from build123d import *

# Parameters (mm, degrees)
F1_DEPTH = 3.175


with BuildPart() as f1:
    # F0 (on Front) → F1 (new body)
    with BuildSketch(Plane.XZ):
        with BuildLine():
            ThreePointArc((18.1003854029, 25.9293170253), (27.7354169074, 14.7579941641), (31.2024073118, 0.4188078519))
            ThreePointArc((31.2024073118, 0.4188078519), (15.6747583451, -26.6663225741), (-15.5443153352, -26.9519992705))
            Line((-15.5443153352, -26.9519992705), (-17.4479872613, -28.6275453194))
            ThreePointArc((-17.4479872613, -28.6275453194), (16.7522947844, -28.9206845921), (33.9376170858, 0.6497384695))
            ThreePointArc((33.9376170858, 0.6497384695), (30.1518596131, 16.2494630696), (19.6368196433, 28.3786551975))
            Line((19.6368196433, 28.3786551975), (18.1003854029, 25.9293170253))
        make_face()
        with BuildLine():
            ThreePointArc((16.3881498341, 27.0734219148), (17.253653438, 26.5154160266), (18.1003854029, 25.9293170253))
            Line((18.1003854029, 25.9293170253), (19.6368196433, 28.3786551975))
            ThreePointArc((19.6368196433, 28.3786551975), (18.8174924383, 28.9438406682), (17.9819876939, 29.4848245007))
            Line((17.9819876939, 29.4848245007), (16.3881498341, 27.0734219148))
        make_face()
        with BuildLine():
            Line((-17.4479872613, -28.6275453194), (-15.5443153352, -26.9519992705))
            ThreePointArc((-15.5443153352, -26.9519992705), (-16.2151958858, -26.5645395925), (-16.8763088681, -26.1606394314))
            Line((-16.8763088681, -26.1606394314), (-18.7192165135, -27.8357967551))
            ThreePointArc((-18.7192165135, -27.8357967551), (-18.0879575097, -28.2386644121), (-17.4479872613, -28.6275453194))
        make_face()
        with BuildLine():
            ThreePointArc((17.9819876939, 29.4848245007), (18.8174924383, 28.9438406682), (19.6368196433, 28.3786551975))
            Line((19.6368196433, 28.3786551975), (33.8907018304, 51.1017739773))
            Line((33.8907018304, 51.1017739773), (14.0615815229, 31.5986632111))
            ThreePointArc((14.0615815229, 31.5986632111), (14.88706319, 31.2075763768), (15.7017518794, 30.7944768319))
            Line((15.7017518794, 30.7944768319), (25.0723678619, 40.2122400701))
            Line((25.0723678619, 40.2122400701), (17.9819876939, 29.4848245007))
        make_face()
        with BuildLine():
            Line((-35.7383415103, -44.7260811925), (-17.4479872613, -28.6275453194))
            ThreePointArc((-17.4479872613, -28.6275453194), (-18.0879575097, -28.2386644121), (-18.7192165135, -27.8357967551))
            Line((-18.7192165135, -27.8357967551), (-27.7228504419, -36.0198765993))
            Line((-27.7228504419, -36.0198765993), (-20.4711550552, -26.6101538588))
            ThreePointArc((-20.4711550552, -26.6101538588), (-21.1322326485, -26.1033010296), (-21.7807070785, -25.5804202701))
            Line((-21.7807070785, -25.5804202701), (-35.7383415103, -44.7260811925))
        make_face()
        with BuildLine():
            ThreePointArc((11.8378918102, 29.4115330659), (12.702739818, 29.0376137231), (13.5559743104, 28.6379030117))
            Line((13.5559743104, 28.6379030117), (15.7017518794, 30.7944768319))
            ThreePointArc((15.7017518794, 30.7944768319), (14.88706319, 31.2075763768), (14.0615815229, 31.5986632111))
            Line((14.0615815229, 31.5986632111), (11.8378918102, 29.4115330659))
        make_face()
        with BuildLine():
            Line((-20.4711550552, -26.6101538588), (-19.0004213571, -24.7017454678))
            ThreePointArc((-19.000421357, -24.7017454678), (-19.6857633723, -24.1734886316), (-20.3562825888, -23.6265398743))
            Line((-20.3562825888, -23.6265398743), (-21.7807070785, -25.5804202701))
            ThreePointArc((-21.7807070785, -25.5804202701), (-21.1322326485, -26.1033010296), (-20.4711550552, -26.6101538588))
        make_face()
        with BuildLine():
            ThreePointArc((-20.3562825888, -23.6265398743), (-27.0142720371, 16.7048556324), (11.8378918102, 29.4115330659))
            Line((11.8378918102, 29.4115330659), (14.0615815229, 31.5986632111))
            ThreePointArc((14.0615815229, 31.5986632111), (-28.9318907936, 18.7255261755), (-21.7807070785, -25.5804202701))
            Line((-21.7807070785, -25.5804202701), (-20.3562825888, -23.6265398743))
        make_face()
        with BuildLine():
            Line((-5.9004323557, 9.0836035088), (13.5559743104, 28.6379030117))
            ThreePointArc((13.5559743104, 28.6379030117), (12.702739818, 29.0376137231), (11.8378918102, 29.4115330659))
            Line((11.8378918102, 29.4115330659), (-11.5615911782, 6.3967597671))
            Line((-11.5615911782, 6.3967597671), (-3.1656639185, 7.3638306931))
            Line((-3.1656639185, 7.3638306931), (-20.9245868027, -14.5271206275))
            Line((-20.9245868027, -14.5271206275), (-12.4407447875, -12.7688115463))
            Line((-12.4407447875, -12.7688115463), (-20.3562825888, -23.6265398743))
            ThreePointArc((-20.3562825888, -23.6265398743), (-19.6857633723, -24.1734886316), (-19.000421357, -24.7017454678))
            Line((-19.0004213571, -24.7017454678), (-7.2250561789, -9.4221569598))
            Line((-7.2250561789, -9.4221569598), (-15.4455099255, -11.0584562644))
            Line((-15.4455099255, -11.0584562644), (1.6187507426, 9.8238335922))
            Line((1.6187507426, 9.8238335922), (-5.9004323557, 9.0836035088))
        make_face()
        with BuildLine():
            Line((14.2855551094, 19.8478270322), (18.1003854029, 25.9293170253))
            ThreePointArc((18.1003854029, 25.9293170253), (17.253653438, 26.5154160266), (16.3881498341, 27.0734219148))
            Line((16.3881498341, 27.0734219148), (10.034003295, 17.4598935992))
            Line((10.034003295, 17.4598935992), (18.7998898327, 17.4598935992))
            Line((18.7998898327, 17.4598935992), (5.6315795518, 0))
            Line((5.6315795518, 0), (11.9040580466, 0))
            Line((11.9040580466, 0), (-16.8763088681, -26.1606394314))
            ThreePointArc((-16.8763088681, -26.1606394314), (-16.2151958858, -26.5645395925), (-15.5443153352, -26.9519992705))
            Line((-15.5443153352, -26.9519992705), (17.4505114555, 2.0889036823))
            Line((17.4505114555, 2.0889036823), (10.2414432913, 2.0889036823))
            Line((10.2414432913, 2.0889036823), (23.1650173664, 19.8478270322))
            Line((23.1650173664, 19.8478270322), (14.2855551094, 19.8478270322))
        make_face()
    extrude(amount=F1_DEPTH)


solid = f1.part
Can you work these out from the model? Positions are in its coordinate system, mm. A direction names the side the tool comes from. Give positions to 0.01 mm unless a question says otherwise; leave off trailing zeros. Loops run counter-clockwise (first coordinate to the right, second up) from the corner with the lowest first, then second, coordinate; pieces in that order, holes last. Notation, with made-up numbers: M -1,57.25 L 44,57.25 A14 ccw 44,80.25 Z; hole C -3.5,-21.5 d6. An arc over 180 degrees is marked long. One line per item, written item: value.
1) On a 3-axis mill with a long thin cutter (end or side, diameter ignored), from which of +Z, -Z, +X, -X, +Y, -Y can I reach the whole of each face in a straight line? I mean faces 1 (the face through (12.308, -1.565, 8.852)), 2 (the face through (-28.66, -1.57, -35.02)). Say none if no direction works.
Geometry check:
face 1: +Y, -Y
face 2: -X, +Y, -Y
2) I'm going to push flat-ended pins straight in: pin 1 (4 mm diameter, centred on x = 19, z = -28.5, fed in from -Y) (3 decimals); pin 2 (1.6 mm diameter, centred on x = 18.5, y = -1, fed in from +Z); pin 3 (1 mm diameter, centred on x = 8, y = -1, fed in from -Z); pin 4 (1 mm diameter, centred on x = 4.5, y = -2, fed in from +Z). Where does each tip first touch, or does it pass through?
Geometry check:
pin 1: stops at y = -3.175
pin 2: stops at z = 36.75
pin 3: stops at z = -32.53
pin 4: stops at z = 34.44
3) Please list where these lines run through material, in increasing order: line 1 (Z direction, x = -5, y = -1.05); line 2 (Z direction, x = 15, y = -0.8); line 3 (X direction, y = -0.3, z = -18).
Geometry check:
line 1: z = -33.03 to -30.6, -17.67 to -15.37, 1.72 to 5.1, 7.15 to 9.17, 9.99 to 12.85, 31.43 to 34.33
line 2: z = -29.85 to -27.05, -0.07 to 2.09, 8.63 to 12.42, 17.46 to 19.85, 20.99 to 24.97, 30.09 to 32.52
line 3: x = -28.56 to -25.6, -16.25 to -13.84, -7.9 to -5.37, 25.23 to 28.37
4) Thinking about a two-plate mould opening in Z: for faces 3 (the face through (-6, 0, 3)), 4 (the face through (26.664, -1.565, 39.581)), 5 (the face through (24.115, -1.565, 41.487)), which applies, +Z half, -Z half, draft (parallel to the pull), parting line (faces both ways), or undercut?
Geometry check:
face 3: draft
face 4: undercut
face 5: +Z half
5) Imagine slicing it at C-C on z = -32. Write out the boundary of the cut face in (x, y) (3 decimals).
Geometry check:
outline: M -26.461,-3.175 L -24.625,-3.175 L -24.625,0 L -26.461,0 Z; M -23.3,-3.175 L -21.28,-3.175 L -21.28,0 L -23.3,0 Z; M -9.701,-3.175 L 9.509,-3.175 L 9.509,0 L -9.701,0 Z
6) Imagine slicing it at B-B on x = -10. Write out the boundary of the cut face in (y, z) (3 decimals).
Geometry check:
outline: M -3.175,-31.91 L 0,-31.91 L 0,-29.393 L -3.175,-29.393 Z; M -3.175,-22.072 L 0,-22.072 L 0,-19.91 L -3.175,-19.91 Z; M -3.175,-13.023 L 0,-13.023 L 0,-9.975 L -3.175,-9.975 Z; M -3.175,-4.395 L 0,-4.395 L 0,-1.061 L -3.175,-1.061 Z; M -3.175,6.577 L 0,6.577 L 0,7.933 L -3.175,7.933 Z; M -3.175,30.231 L 0,30.231 L 0,33.21 L -3.175,33.21 Z
7) Imagine slicing it at A-A on x = 27.5. Write out the boundary of the cut face in (y, z) (3 decimals).
Geometry check:
outline: M -3.175,-19.269 L 0,-19.269 L 0,-14.37 L -3.175,-14.37 Z; M -3.175,15.207 L 0,15.207 L 0,20.568 L -3.175,20.568 Z; M -3.175,40.914 L 0,40.914 L 0,44.816 L -3.175,44.816 Z
